```python
from build123d import *

# Parameters (mm, degrees)
BOSS_EXTRUDE1_DEPTH = 3
CHAMFER1_SIZE       = 0.5


with BuildPart() as part:
    # Sketch1 → Boss-Extrude1 (new, symmetric)
    with BuildSketch(Plane(origin=(0, 0, 0), x_dir=(1, 0, 0), z_dir=(0, 1, 0))):
        Polygon((-4.674503569, 1.610851049), (-1.08284245, 1.547271789), (0.087509344, 4.943497429), (1.136926198, 1.507977646), (4.728587318, 1.444398386), (1.785501483, -0.61529035), (2.834918338, -4.050810134), (-0.033425595, -1.888247995), (-2.97651143, -3.94793673), (-1.806159637, -0.55171109), align=None)
    extrude(amount=BOSS_EXTRUDE1_DEPTH, both=True)

    # Chamfer1
    chamfer1_edges = [part.edges().sort_by_distance(p)[0] for p in [
        (0.612217771, -3, -3.225737537),
        (2.932756758, -3, -1.476188016),
        (3.2570444, -3, -0.414554018),
        (2.31020991, -3, 2.333050242),
        (1.400746371, -3, 2.969529064),
        (-1.504968513, -3, 2.918092363),
        (-2.391335533, -3, 2.24982391),
        (-3.240331603, 3, -0.529569979),
        (-3.240331603, -3, -0.529569979),
        (-2.878673009, -3, -1.579061419),
        (-0.497666553, -3, -3.245384609),
        (-2.391335533, 3, 2.24982391),
        (-1.504968513, 3, 2.918092363),
        (1.400746371, 3, 2.969529064),
        (2.31020991, 3, 2.333050242),
        (3.2570444, 3, -0.414554018),
        (2.932756758, 3, -1.476188016),
        (0.612217771, 3, -3.225737537),
        (-0.497666553, 3, -3.245384609),
        (-2.878673009, 3, -1.579061419),
    ]]
    chamfer(chamfer1_edges, length=CHAMFER1_SIZE)


solid = part.part
```
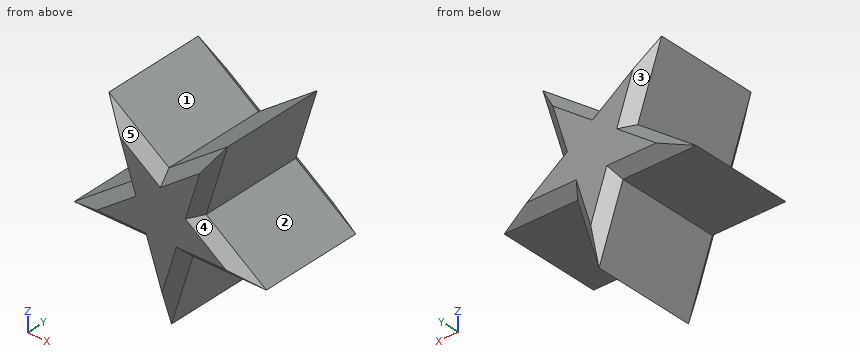
Design review of the part built by this model. Coordinates are the model's own, in mm. Face numbers are marked on the shaded views. A direction names the side the tool comes from. Coordinates: 2 decimals unless noted, no trailing zeros. Loops run counter-clockwise (first coordinate to the right, second up) from the corner with the lowest first, then second, coordinate; pieces in that order, holes last.
Q1. We need section D-D on x = 0.25. State the section outline as (y, z) points.
Reported:
outline: (-3, -2.7) - (-2.5, -4.41) - (2.5, -4.41) - (3, -2.7) - (3, 1.48) - (2.5, 2.1) - (-2.5, 2.1) - (-3, 1.48) - close
Q2. To check wall thickness, follow line 1 (X direction, y = 2, z = 2); line 2 (X direction, y = 2, z = 2.5); line 3 (Z direction, x = -1.25, y = 0.75). State the ranges of each line that lie inside material, in increasing order.
Reported:
line 1: x = -2.31 to -0.19, 0.11 to 2.21
line 2: x = -2.48 to -0.91, 0.78 to 2.36
line 3: z = -1.55 to 2.74
Q3. Tool access review of the marked faces 1, 2, 3, 4 and 5: name each direction out of +Z, -Z, +X, -X, +Y, -Y from which nothing blocks a thin tool from reaching the whole face with its end or side.
Reported:
face 1: +Z, +Y, -Y
face 2: +X, +Y, -Y
face 3: -X, +Y
face 4: +X, -Y
face 5: +Z, -Y
Q4. We need section C-C on z = -0.25. State the section outline as (x, y) points.
Reported:
outline: (-2.87, -2.5) - (-2.04, -3) - (2.15, -3) - (3.02, -2.5) - (3.02, 2.5) - (2.15, 3) - (-2.04, 3) - (-2.87, 2.5) - close
Q5. For pin 1 (1.5 mm diameter, centred on y = 2, z = 0, fed in from +X); pin 2 (3 mm diameter, centred on y = 2, z = 0.5, fed in from -X); pin 3 (3 mm diameter, centred on x = 1.5, y = -2, fed in from +Z), all flat-tipped, find the tip position at first contact; note any pin that passes through.
Reported:
pin 1: stops at x = 3.74
pin 2: stops at x = -3.86
pin 3: stops at z = 4.05
Q6. We need section A-A on y = -1.5. State the section outline as (x, z) points, and give its area (3 significant figures).
Reported:
outline: (-4.67, -1.61) - (-1.08, -1.55) - (0.09, -4.94) - (1.14, -1.51) - (4.73, -1.44) - (1.79, 0.62) - (2.83, 4.05) - (-0.03, 1.89) - (-2.98, 3.95) - (-1.81, 0.55) - close
area: 27.4 mm2
Q7. We need section B-B on z = 2.5. State the section outline as (x, y) points.
Reported:
outline: (-2.48, -2.5) - (-1.95, -3) - (-1.78, -3) - (-0.91, -2.5) - (-0.91, 2.5) - (-1.78, 3) - (-1.95, 3) - (-2.48, 2.5) - close; (0.78, -2.5) - (1.61, -3) - (1.84, -3) - (2.36, -2.5) - (2.36, 2.5) - (1.84, 3) - (1.61, 3) - (0.78, 2.5) - close
